Geometry check sheet. Reference: the model listing, model coordinates, mm. A direction names the side the tool comes from. Give positions to 0.01 mm unless a question says otherwise; leave off trailing zeros. Loops run counter-clockwise (first coordinate to the right, second up) from the corner with the lowest first, then second, coordinate; pieces in that order, holes last. Notation, with made-up numbers: (2.5, 10.5) -> (39.5, 10.5) arc R26 cw to (39.5, 26.5) -> close; hole circle Ø10 at (19, 46.5). An arc over 180 degrees is marked (long way). Write item = value, one per line. Start each with the question number.
```python
from build123d import *

# Parameters (mm, degrees)
SKETCH1_W           = 55.7
SKETCH1_H           = 31.7
BOSS_EXTRUDE1_DEPTH = 16
SKETCH3_W           = 51.7
SKETCH3_H           = 27.7
CUT_EXTRUDE2_DEPTH  = 15
CUT_EXTRUDE3_START  = -5
SKETCH4_W           = 13.581579568
SKETCH4_H           = 13.316801047
CUT_EXTRUDE3_DEPTH  = 21
SKETCH5_W           = 7.7
SKETCH5_H           = 6
CUT_EXTRUDE4_DEPTH  = 10
SKETCH7_W           = 13.7
SKETCH7_H           = 14.99631632
CUT_EXTRUDE5_DEPTH  = 10


with BuildPart() as part:
    # Sketch1 → Boss-Extrude1 (new body)
    with BuildSketch(Plane(origin=(0, 0, 0), x_dir=(1, 0, 0), z_dir=(0, 1, 0))):
        with Locations((27.85, 15.85)):
            Rectangle(SKETCH1_W, SKETCH1_H)
    extrude(amount=BOSS_EXTRUDE1_DEPTH)

    # Sketch3 → Cut-Extrude2 (cut)
    with BuildSketch(Plane.XZ):
        with Locations((27.85, -15.85)):
            Rectangle(SKETCH3_W, SKETCH3_H)
    extrude(amount=-CUT_EXTRUDE2_DEPTH, mode=Mode.SUBTRACT)

    # Sketch4 → Cut-Extrude3 (cut, through all)
    with BuildSketch(Plane.XZ.offset(-15).offset(CUT_EXTRUDE3_START)):
        with Locations((27.790789784, -5.841599476)):
            Rectangle(SKETCH4_W, SKETCH4_H)
    extrude(amount=CUT_EXTRUDE3_DEPTH, mode=Mode.SUBTRACT)

    # Sketch5 → Cut-Extrude4 (cut)
    with BuildSketch(Plane.XZ.offset(-15)):
        with Locations((27.85, -22.7)):
            Rectangle(SKETCH5_W, SKETCH5_H)
    extrude(amount=-CUT_EXTRUDE4_DEPTH, mode=Mode.SUBTRACT)

    # Sketch7 → Cut-Extrude5 (cut)
    with BuildSketch(Plane.ZY):
        with Locations((-15.85, 6.784922937)):
            Rectangle(SKETCH7_W, SKETCH7_H)
    extrude(amount=-CUT_EXTRUDE5_DEPTH, mode=Mode.SUBTRACT)


solid = part.part
```
1) Section check B-B (z = -10). Enter the section's corners in (x, y), plus the area to 3 significant figures.
2) Section check C-C (x = 30). Enter the section's corners in (y, z), plus the area to 3 significant figures.
3) Thickness scan on line 1 (Z direction, x = 41.5, y = 10.75); line 2 (X direction, y = 7, z = -6.5); line 3 (Z direction, x = 27, y = 9). Record the ranges inside material, lowest first.
4) Depth check by flat-ended pin: pin 1 Ø3 at (x, z) = (33, -13) entering from -Y; pin 2 Ø3 at (y, z) = (4.5, -20) entering from -X; pin 3 Ø0.5 at (x, y) = (25, 15.5) entering from +Z. Enter the tip coordinate at first touch or a pass-through.
5) Section check D-D (z = -24). Enter the section's corners in (x, y), plus the area to 3 significant figures.
6) Draft check along X on faces 5 (the flat face through (10, 8, 0)), 6 (the flat face through (27.7, 15.5, -12.5)), 7 (the flat face through (55.7, 8, -16)). Enter one of: released by +X, released by -X, zero draft, split by the parting line, or undercut.
7) Tool access check on faces 1 (the flat face through (1, 7, -22.7)), 2 (the flat face through (2, 7, -25)), 3 (the flat face through (21, 10.4, -1.6)), 4 (the flat face through (24, 15.5, -22.7)). Record the directions out of +Z, -Z, +X, -X, +Y, -Y that give a thin tool (end or side, any length) a straight path to the whole face; none if there is none.
8) Section check A-A (y = 2). Enter the section's corners in (x, z), plus the area to 3 significant figures.
Check result:
q1.outline = (0, 14.28) -> (2, 14.28) -> (2, 15) -> (21, 15) -> (21, 16) -> (0, 16) -> close; (34.58, 15) -> (53.7, 15) -> (53.7, 0) -> (55.7, 0) -> (55.7, 16) -> (34.58, 16) -> close
q1.area = 73.6 mm2
q2.outline = (0, -31.7) -> (16, -31.7) -> (16, -25.7) -> (15, -25.7) -> (15, -29.7) -> (0, -29.7) -> close; (15, -19.7) -> (16, -19.7) -> (16, -12.5) -> (15, -12.5) -> close
q2.area = 43.2 mm2
q3.line_1 = -31.7 to -29.7, -2 to 0
q3.line_2 = 0 to 2, 53.7 to 55.7
q3.line_3 = -31.7 to -29.7
q4.pin_1 = 15
q4.pin_2 = 53.7
q4.pin_3 = -12.5
q5.outline = (0, 0) -> (2, 0) -> (2, 15) -> (24, 15) -> (24, 16) -> (0, 16) -> close; (31.7, 15) -> (53.7, 15) -> (53.7, 0) -> (55.7, 0) -> (55.7, 16) -> (31.7, 16) -> close
q5.area = 108 mm2
q6.face_5 = zero draft
q6.face_6 = undercut
q6.face_7 = released by +X
q7.face_1 = -X, -Y
q7.face_2 = -Y
q7.face_3 = +Z, +Y, -Y
q7.face_4 = +Y, -Y
q8.outline = (0, -31.7) -> (55.7, -31.7) -> (55.7, 0) -> (34.58, 0) -> (34.58, -2) -> (53.7, -2) -> (53.7, -29.7) -> (2, -29.7) -> (2, -22.7) -> (0, -22.7) -> close; (0, -9) -> (2, -9) -> (2, -2) -> (21, -2) -> (21, 0) -> (0, 0) -> close
q8.area = 279 mm2
